Source: CAD feature listing. Evaluate the final solid. Frame: model axes, mm. A direction names the side the tool comes from. Round coordinates to 2 decimals unless told otherwise and drop trailing zeros. Order: outer loops, then holes, each group sorted by start corner. A loop starts at its lowest first (then second) coordinate and runs counter-clockwise, first axis right, second up. Notation, with made-up numbers: M -35.75,-25.75 L -28.75,-25.75 A32 cw -28.75,10.25 Z; hole C 76,-10 d10. An arc over 180 degrees is marked long. Answer as CSV lines item,"result". Start each with the question number.
Item 1: Section query B-B on z = 8. Return the cut outline in (x, y), plus the area to 3 significant figures.
Item 2: Section query C-C on z = 1.5. Return the cut outline in (x, y).
Item 3: Set-up query: faces 5 (the face through (21, 3, 4)), 6 (the face through (31.1, 1.48, 16.64)). Return all of +Z, -Z, +X, -X, +Y, -Y with unobstructed straight access to the full face (end or side cutting, diameter ignored); none if empty.
Item 4: First-contact query: P1, Ø5, axis at x = 18, z = 9, coming from the -Y side; P2, Ø3, axis at x = 10, z = 11, coming from the +Y side; P3, Ø10.5, axis at y = 28.5, z = 2.5, coming from the +X side. Flat tips, straight axial feed; report the tip coordinate or a pass-through.
Item 5: Line query: line 1 (Z direction, x = 1, y = 20); line 2 (X direction, y = 1, z = 8); line 3 (Y direction, x = 12.5, z = 13.5). Output: solid intervals per line, ascending. Write a range as [from, to].
Item 6: Pull-direction query (X, two-part tool) for faces 1 (the face through (0, 22, 0)), 2 (the face through (24.586, 1.521, -8.208)), 3 (the face through (2, 19, -13)), 4 (the face through (32, 2, 0)); classes: +X half, -X half, draft (parallel to the pull), parting line (faces both ways), or undercut.
Item 7: Section query D-D on y = 16.5. Return the cut outline in (x, z), plus the area to 3 significant figures.
Item 8: Section query A-A on x = 23. Return the cut outline in (y, z).
from build123d import *

# Parameters (mm, degrees)
EXTRUDE_1_DEPTH     = 17.5
SKETCH_2_R          = 1.6
CUT_EXTRUDE_2_DEPTH = 26
SKETCH_3_R          = 5
SKETCH_3_R_2        = 1.6
CUT_EXTRUDE_3_DEPTH = 56.625983137
FILLET_2_R          = 3


with BuildPart() as part:
    # 草图1 → 凸台-拉伸1 (new, symmetric)
    with BuildSketch(Plane.XY):
        Polygon((0, 0), (0, 45), (3, 45), (3, 3), (32, 3), (32, 0), align=None)
    extrude(amount=EXTRUDE_1_DEPTH, both=True)

    # 草图2 → 切除-拉伸2 (cut)
    with BuildSketch(Plane(origin=(3, 0, 0), x_dir=(0, 0, -1), z_dir=(1, 0, 0))):
        with BuildLine():
            Line((17.5, 27.5), (17.5, 45))
            Line((17.5, 45), (3.9e-08, 45))
            ThreePointArc((3.9e-08, 45), (12.374368684, 39.874368657), (17.5, 27.5))
        make_face()
        with BuildLine():
            ThreePointArc((-17.5, 27.5), (-12.374368657, 39.874368684), (3.9e-08, 45))
            Line((3.9e-08, 45), (-17.5, 45))
            Line((-17.5, 45), (-17.5, 27.5))
        make_face()
        with Locations(Location((-11.75, 20, 0), (0, 0, 90))):
            Circle(SKETCH_2_R)
        with Locations(Location((11.75, 20, 0), (0, 0, 90))):
            Circle(SKETCH_2_R)
        with Locations(Location((-11.75, 32.09, 0), (0, 0, 90))):
            Circle(SKETCH_2_R)
        with Locations(Location((11.75, 32.09, 0), (0, 0, 90))):
            Circle(SKETCH_2_R)
    extrude(amount=-CUT_EXTRUDE_2_DEPTH, mode=Mode.SUBTRACT)

    # 草图3 → 切除-拉伸3 (cut, through all)
    with BuildSketch(Plane(origin=(0, 3, 0), x_dir=(1, 0, 0), z_dir=(0, 1, 0))):
        with Locations(Location((16, 0, 0), (0, 0, 270))):
            Circle(SKETCH_3_R)
        with Locations(Location((9, 8, 0), (0, 0, 270))):
            Circle(SKETCH_3_R_2)
        with Locations(Location((23, 8, 0), (0, 0, 270))):
            Circle(SKETCH_3_R_2)
        with Locations(Location((23, -8, 0), (0, 0, 270))):
            Circle(SKETCH_3_R_2)
        with Locations(Location((9, -8, 0), (0, 0, 270))):
            Circle(SKETCH_3_R_2)
    extrude(amount=-CUT_EXTRUDE_3_DEPTH, mode=Mode.SUBTRACT)

    # 圆角2
    fillet_2_edges = [part.edges().sort_by_distance(p)[0] for p in [
        (32, 1.5, -17.5),
        (32, 1.5, 17.5),
    ]]
    fillet(fillet_2_edges, radius=FILLET_2_R)


solid = part.part
Results:
1,outline,"M 0,0 L 7.4,0 L 7.4,3 L 3,3 L 3,43.06 L 0,43.06 Z; M 10.6,0 L 21.4,0 L 21.4,3 L 10.6,3 Z; M 24.6,0 L 32,0 L 32,3 L 24.6,3 Z"
1,area,"197 mm^2"
2,outline,"M 0,0 L 11.23,0 L 11.23,3 L 3,3 L 3,44.94 L 0,44.94 Z; M 20.77,0 L 32,0 L 32,3 L 20.77,3 Z"
3,face 5,"+Z, -Z, +X, +Y"
3,face 6,"+Z, +X, +Y, -Y"
4,P1,"y = 0"
4,P2,"y = 3"
4,P3,"x = 3"
5,line 1,"[-17.5, -13.35], [-10.15, 10.15], [13.35, 17.5]"
5,line 2,"[0, 7.4], [10.6, 21.4], [24.6, 32]"
5,line 3,"[0, 3]"
6,face 1,"-X half"
6,face 2,"undercut"
6,face 3,"draft"
6,face 4,"+X half"
7,outline,"M 0,-17.5 L 3,-17.5 L 3,17.5 L 0,17.5 Z"
7,area,"105 mm^2"
8,outline,"M 0,-17.5 L 3,-17.5 L 3,-9.6 L 0,-9.6 Z; M 0,-6.4 L 3,-6.4 L 3,6.4 L 0,6.4 Z; M 0,9.6 L 3,9.6 L 3,17.5 L 0,17.5 Z"
